CAD build for the part. Positions are in the model's coordinates, mm. Face numbers are marked on the shaded views. Give positions to 0.01 mm unless a question says otherwise; leave off trailing zeros. Loops run counter-clockwise (first coordinate to the right, second up) from the corner with the lowest first, then second, coordinate; pieces in that order, holes last.
Item 1: Probe probe 1 along X at (y, z) = (-4.4, 5); probe 2 along Z at (x, y) = (11, -2.85); probe 3 along X at (y, z) = (-1.85, 5). List the from-to ranges inside material, lowest first.
Item 2: Mould opens along X. For the marked faces 1, 2 and 3 say: released by +X, released by -X, zero draft, split by the parting line, or undercut.
Item 3: Saw through at C-C on x = 11. Give the cut face in (y, z), plus the area to 4 significant figures.
Item 4: Saw through at A-A on y = -0.8. Give the cut face in (x, z).
Item 5: Saw through at B-B on z = 9.5. Give the cut face in (x, y) (3 decimals).
Item 6: Drop flat-ended pins along their axis: P1, Ø3, axis at y = -2, z = 6, coming from the -X side; P2, Ø1.5, axis at y = -2, z = 1.5, coming from the -X side. Give the stop position or say it passes through.
Item 7: Saw through at D-D on z = 4.25. Give the cut face in (x, y) (3 decimals), plus the area to 3 significant figures.
from build123d import *

# Parameters (mm, degrees)
SKETCH1_W           = 30
SKETCH1_H           = 11
SKETCH1_R           = 4
BOSS_EXTRUDE1_DEPTH = 10
SKETCH2_R           = 1.5
CUT_EXTRUDE1_DEPTH  = 17
CUT_EXTRUDE2_START  = -17
CUT_EXTRUDE2_DEPTH  = 17
CUT_EXTRUDE3_DEPTH  = 17


with BuildPart() as part:
    # Sketch1 → Boss-Extrude1 (new body)
    with BuildSketch(Plane.XY):
        Rectangle(SKETCH1_W, SKETCH1_H)
        Circle(SKETCH1_R, mode=Mode.SUBTRACT)
    extrude(amount=BOSS_EXTRUDE1_DEPTH)

    # Sketch2 → Cut-Extrude1 (cut)
    with BuildSketch(Plane(origin=(0, 5.5, 0), x_dir=(1, 0, 0), z_dir=(0, 1, 0))):
        with Locations(Location((-11, -5, 0), (0, 0, 270))):
            Circle(SKETCH2_R)
        with Locations(Location((11, -5, 0), (0, 0, 270))):
            Circle(SKETCH2_R)
    extrude(amount=-CUT_EXTRUDE1_DEPTH, mode=Mode.SUBTRACT)

    # Sketch3 → Cut-Extrude2 (cut)
    with BuildSketch(Plane.XY.offset(10).offset(CUT_EXTRUDE2_START)):
        with BuildLine():
            Line((3.992179856, -0.25), (15, -0.25))
            Line((15, -0.25), (15, 5.5))
            Line((15, 5.5), (-15, 5.5))
            Line((-15, 5.5), (-15, -0.25))
            Line((-15, -0.25), (-3.992179856, -0.25))
            ThreePointArc((-3.992179856, -0.25), (0, 4), (3.992179856, -0.25))
        make_face()
    extrude(amount=CUT_EXTRUDE2_DEPTH, mode=Mode.SUBTRACT)

    # Sketch4 → Cut-Extrude3 (cut)
    with BuildSketch(Plane.XY.offset(10)):
        Polygon((-15, -2.875), (-12.5, -0.25), (-15, -0.25), align=None)
        Polygon((15, -0.25), (12.5, -0.25), (15, -2.875), align=None)
    extrude(amount=-CUT_EXTRUDE3_DEPTH, mode=Mode.SUBTRACT)


solid = part.part
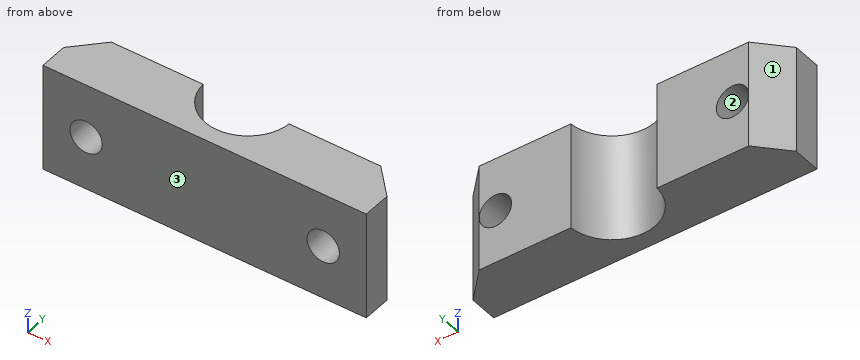
Results below:
1. probe 1: x = -15 to -12.5, -9.5 to 9.5, 12.5 to 15
1. probe 2: z = 0 to 3.5, 6.5 to 10
1. probe 3: x = -14.02 to -12.5, -9.5 to -3.55, 3.55 to 9.5, 12.5 to 14.02
2. face 1: released by -X
2. face 2: undercut
2. face 3: zero draft
3. outline: (-5.5, 0) - (-0.25, 0) - (-0.25, 3.5) - (-5.5, 3.5) - close; (-5.5, 6.5) - (-0.25, 6.5) - (-0.25, 10) - (-5.5, 10) - close
3. area: 36.75 mm2
4. outline: (-13.02, 0) - (-3.92, 0) - (-3.92, 10) - (-13.02, 10) - close; (3.92, 0) - (13.02, 0) - (13.02, 10) - (3.92, 10) - close; hole circle Ø3 at (-11, 5); hole circle Ø3 at (11, 5)
5. outline: (-15, -5.5) - (15, -5.5) - (15, -2.875) - (12.5, -0.25) - (3.992, -0.25) arc R4 cw to (-3.992, -0.25) - (-12.5, -0.25) - (-15, -2.875) - close
6. P1: stops at x = -15
6. P2: stops at x = -14.88
7. outline: (-15, -5.5) - (-12.299, -5.5) - (-12.299, -0.25) - (-12.5, -0.25) - (-15, -2.875) - close; (-9.701, -5.5) - (9.701, -5.5) - (9.701, -0.25) - (3.992, -0.25) arc R4 cw to (-3.992, -0.25) - (-9.701, -0.25) - close; (12.299, -5.5) - (15, -5.5) - (15, -2.875) - (12.5, -0.25) - (12.299, -0.25) - close
7. area: 101 mm2
